from build123d import *

# Parameters (mm, degrees)
ESQUISSE1_W        = 80
ESQUISSE1_H        = 80
ESQUISSE1_R        = 2
BOSS_EXTRU_1_DEPTH = 1.16
ESQUISSE2_W        = 28.5
ESQUISSE2_H        = 16.5
BOSS_EXTRU_2_DEPTH = 17.3
ESQUISSE3_W        = 9.5
ESQUISSE3_H        = 3.65
ESQUISSE3_W_2      = 3.65
ESQUISSE3_H_2      = 9.5
ESQUISSE3_W_3      = 5
ESQUISSE3_H_3      = 6.35
BOSS_EXTRU_3_DEPTH = 6


with BuildPart() as part:
    # Esquisse1 → Boss.-Extru.1 (new body)
    with BuildSketch(Plane(origin=(0, 0, 0), x_dir=(1, 0, 0), z_dir=(0, 1, 0))):
        Rectangle(ESQUISSE1_W, ESQUISSE1_H)
        with Locations(Location((-35.94, 35.94, 0), (0, 0, 270))):
            Circle(ESQUISSE1_R, mode=Mode.SUBTRACT)
        with Locations(Location((19.58, 35.94, 0), (0, 0, 270))):
            Circle(ESQUISSE1_R, mode=Mode.SUBTRACT)
        with Locations(Location((35.94, -27.79, 0), (0, 0, 270))):
            Circle(ESQUISSE1_R, mode=Mode.SUBTRACT)
        with Locations(Location((-21.64, -36.03, 0), (0, 0, 270))):
            Circle(ESQUISSE1_R, mode=Mode.SUBTRACT)
    extrude(amount=BOSS_EXTRU_1_DEPTH)

    # Esquisse2 → Boss.-Extru.2 (add)
    with BuildSketch(Plane(origin=(0, 1.16, 0), x_dir=(1, 0, 0), z_dir=(0, 1, 0))):
        with Locations((6.65, 11.55)):
            Rectangle(ESQUISSE2_W, ESQUISSE2_H)
        with Locations((6.65, -11.45)):
            Rectangle(ESQUISSE2_W, ESQUISSE2_H)
    extrude(amount=BOSS_EXTRU_2_DEPTH)

    # Esquisse3 → Boss.-Extru.3 (add)
    with BuildSketch(Plane.XZ):
        with Locations((33.53, 36.975)):
            Rectangle(ESQUISSE3_W, ESQUISSE3_H)
        with Locations((15.17, 36.975)):
            Rectangle(ESQUISSE3_W, ESQUISSE3_H)
        with Locations((-3.53, 36.975)):
            Rectangle(ESQUISSE3_W, ESQUISSE3_H)
        with Locations((3.275, -12.45)):
            Rectangle(ESQUISSE3_W_2, ESQUISSE3_H_2)
        with Locations((-36.975, -19.75)):
            Rectangle(ESQUISSE3_W_2, ESQUISSE3_H_2)
        with Locations((-13, -8.225)):
            Rectangle(ESQUISSE3_W_3, ESQUISSE3_H_3)
    extrude(amount=BOSS_EXTRU_3_DEPTH)


solid = part.part
Input: part model. Units: mm. Frame: model coordinates. A direction names the side the tool comes from. Round coordinates to 2 decimals unless told otherwise and drop trailing zeros. Write each loop counter-clockwise with the first axis right and the second up, starting at its lowest first coordinate (ties: lowest second). Pieces come first, ordered by that corner, then holes.
1) Cut plane C-C (z = -35.94). Return the cut outline in (x, y), then the cut area to 3 significant figures.
2) Cut plane A-A (x = 35.94). Return the cut outline in (y, z), then the cut area to 3 significant figures.
3) Ray query, L1, parallel to X at y = 0.3, z = -35.94; L2, parallel to Z at x = 1.5, y = 15; L3, parallel to X at y = 0.75, z = 36.03. Return the intervals inside material, ascending.
4) Cut plane B-B (y = 6.5). Return the cut outline in (x, z), then the cut area to 4 significant figures.
5) Cut plane D-D (z = 27.79). Return the cut outline in (x, y).
6) Contact query for flat-ended pins moving along their axis: P1, Ø1.5, axis at y = 3.5, z = 1, coming from the +X side; P2, Ø2, axis at x = -6.5, z = -24, coming from the -Y side; P3, Ø4, axis at x = -19, z = -31.5, coming from the +Y side; P4, Ø1.1, axis at y = -4.5, z = 36, coming from the +X side. Output: stop coordinate, or through.
7) Draft query along X for faces 6 (the flat face through (38.28, -3, 37)), 7 (the flat face through (15, -3, 38.8)), 8 (the flat face through (19.92, -3, 37)), 9 (the flat face through (-8.28, -3, 37)). Return one class per face: pulls with the +X half, pulls with the -X half, needs draft (parallel to the pull), parting line crosses it, or undercut.
8) Reachability of faces 1 (the flat face through (3, -3, -7.7)), 2 (the flat face through (6, 10, 3.2)), 3 (the flat face through (-37, -3, -24.5)), 4 (the flat face through (6, 10, 19.7)), 5 (the flat face through (28.78, -3, 37)) from +Z, -Z, +X, -X, +Y, -Y: full face, straight path, thin tool, end or side. Return the list, or none.
Geometry says:
1. outline: (-40, 0) - (-37.94, 0) - (-37.94, 1.16) - (-40, 1.16) - close; (-33.94, 0) - (17.58, 0) - (17.58, 1.16) - (-33.94, 1.16) - close; (21.58, 0) - (40, 0) - (40, 1.16) - (21.58, 1.16) - close
1. area: 83.5 mm2
2. outline: (-6, 35.15) - (0, 35.15) - (0, 29.79) - (1.16, 29.79) - (1.16, 40) - (0, 40) - (0, 38.8) - (-6, 38.8) - close; (0, -40) - (1.16, -40) - (1.16, 25.79) - (0, 25.79) - close
2. area: 110 mm2
3. L1: x = -40 to -37.94, -33.94 to 17.58, 21.58 to 40
3. L2: z = -19.8 to -3.3, 3.2 to 19.7
3. L3: x = -40 to -23.64, -19.64 to 40
4. outline: (-7.6, -19.8) - (20.9, -19.8) - (20.9, -3.3) - (-7.6, -3.3) - close; (-7.6, 3.2) - (20.9, 3.2) - (20.9, 19.7) - (-7.6, 19.7) - close
4. area: 940.5 mm2
5. outline: (-40, 0) - (33.94, 0) - (33.94, 1.16) - (-40, 1.16) - close; (37.94, 0) - (40, 0) - (40, 1.16) - (37.94, 1.16) - close
6. P1: passes through
6. P2: stops at y = 0
6. P3: stops at y = 1.16
6. P4: stops at x = 38.28
7. face 6: pulls with the +X half
7. face 7: needs draft
7. face 8: undercut
7. face 9: pulls with the -X half
8. face 1: +Z, +X, -Y
8. face 2: +X, -X, +Y
8. face 3: -Z, +X, -X, -Y
8. face 4: +Z, +X, -X, +Y
8. face 5: +Z, -Z, -Y
